Part model, mm, in its own coordinate system. A direction names the side the tool comes from. Round coordinates to 2 decimals unless told otherwise and drop trailing zeros. Write each loop counter-clockwise with the first axis right and the second up, starting at its lowest first coordinate (ties: lowest second). Pieces come first, ordered by that corner, then holes.
```python
from build123d import *

# Parameters (mm, degrees)
BOSS_EXTRUDE1_DEPTH        = 20
SKETCH2_W                  = 22.6
SKETCH2_H                  = 12.7
CUT_EXTRUDE1_DEPTH         = 10
F_2_CLEARANCE_HOLE1_REACH  = 69.082
F_2_CLEARANCE_HOLE1_BORE_R = 1.2192


with BuildPart() as part:
    # Sketch1 → Boss-Extrude1 (new body)
    with BuildSketch(Plane.XY):
        Polygon((1.59, -50), (1.59, -1.59), (38.41, -1.59), (38.41, -50), (40, -50), (40, 0), (0, 0), (0, -50), align=None)
    extrude(amount=BOSS_EXTRUDE1_DEPTH)

    # Sketch2 → Cut-Extrude1 (cut)
    with BuildSketch(Plane(origin=(0, 0, 0), x_dir=(1, 0, 0), z_dir=(0, 1, 0))):
        with Locations((20, -6.35)):
            Rectangle(SKETCH2_W, SKETCH2_H)
    extrude(amount=-CUT_EXTRUDE1_DEPTH, mode=Mode.SUBTRACT)

    # #2 Clearance Hole1 bore → #2 Clearance Hole1 (cut, up to next)
    with BuildSketch(Plane.ZY, mode=Mode.PRIVATE) as f_2_clearance_hole1_sk1:
        with Locations((2.5, -5)):
            Circle(F_2_CLEARANCE_HOLE1_BORE_R)
    f_2_clearance_hole1_tool1 = extrude(f_2_clearance_hole1_sk1.sketch, amount=-F_2_CLEARANCE_HOLE1_REACH, mode=Mode.PRIVATE) & part.part
    # #2 Clearance Hole1 bore → #2 Clearance Hole1 (cut, up to next)
    with BuildSketch(Plane.ZY, mode=Mode.PRIVATE) as f_2_clearance_hole1_sk2:
        with Locations((17.5, -45)):
            Circle(F_2_CLEARANCE_HOLE1_BORE_R)
    f_2_clearance_hole1_tool2 = extrude(f_2_clearance_hole1_sk2.sketch, amount=-F_2_CLEARANCE_HOLE1_REACH, mode=Mode.PRIVATE) & part.part
    add(f_2_clearance_hole1_tool1.solids().sort_by_distance((0, -5, 2.5))[0], mode=Mode.SUBTRACT)
    add(f_2_clearance_hole1_tool2.solids().sort_by_distance((0, -45, 17.5))[0], mode=Mode.SUBTRACT)


solid = part.part
```
Q1. Cut at C-C on z = 2.5. Write the cut outline in (x, y), plus the area to 3 significant figures.
Values follow:
outline: (0, -50) - (1.59, -50) - (1.59, -6.22) - (0, -6.22) - close; (0, -3.78) - (1.59, -3.78) - (1.59, -1.59) - (8.7, -1.59) - (8.7, 0) - (0, 0) - close; (31.3, -1.59) - (38.41, -1.59) - (38.41, -50) - (40, -50) - (40, 0) - (31.3, 0) - close
area: 178 mm2
Q2. Mould opens along X. For faces 4 (the flat face through (1.59, -26, 10)), 5 (the flat face through (40, -25, 10)), 6 (the flat face through (31.3, -1, 6)), 7 (the flat face through (1, -50, 10)) say: +X half, -X half, draft (parallel to the pull), parting line (faces both ways), or undercut.
Values follow:
face 4: undercut
face 5: +X half
face 6: undercut
face 7: draft
Q3. Drop flat-ended pins along their axis: pin 1 (2 mm diameter, centred on y = -45, z = 17.5, fed in from -X); pin 2 (10 mm diameter, centred on x = 21, z = 4, fed in from -Y); pin 3 (1.7 mm diameter, centred on x = 16.5, y = -1, fed in from -Z); pin 4 (10 mm diameter, centred on x = 14.5, z = 9.5, fed in from -Y). Give the stop position or say it passes through.
Values follow:
pin 1: stops at x = 38.41
pin 2: passes through
pin 3: stops at z = 12.7
pin 4: stops at y = -1.59
Q4. Cut at D-D on z = 6.75. Write the cut outline in (x, y), plus the area to 3 significant figures.
Values follow:
outline: (0, -50) - (1.59, -50) - (1.59, -1.59) - (8.7, -1.59) - (8.7, 0) - (0, 0) - close; (31.3, -1.59) - (38.41, -1.59) - (38.41, -50) - (40, -50) - (40, 0) - (31.3, 0) - close
area: 182 mm2
Q5. Which spindle directions (+Z, -Z, +X, -X, +Y, -Y) get a long thin tool onto all of the face, cutting with end or side? Do faces 1 (the cylindrical face through (0.78, -44.18, 16.6)), 2 (the flat face through (38.41, -25, 10)), 3 (the flat face through (20, -1, 12.7)). Say none if no direction does.
Values follow:
face 1: -X
face 2: +Z, -Z, -Y
face 3: -Z, +Y, -Y
Q6. Cut at A-A on z = 17.5. Write the cut outline in (x, y), plus the area to 3 significant figures.
Values follow:
outline: (0, -50) - (1.59, -50) - (1.59, -46.22) - (0, -46.22) - close; (0, -43.78) - (1.59, -43.78) - (1.59, -1.59) - (38.41, -1.59) - (38.41, -50) - (40, -50) - (40, 0) - (0, 0) - close
area: 214 mm2
Q7. Wall check: L1, parallel to Y at x = 0.55, z = 2.5; L2, parallel to Y at x = 1.2, z = 17.5; L3, parallel to X at y = -44.5, z = 19. Give the ranges that are in metal, low to high.
Values follow:
L1: y = -50 to -6.22, -3.78 to 0
L2: y = -50 to -46.22, -43.78 to 0
L3: x = 0 to 1.59, 38.41 to 40
Q8. Cut at B-B on y = -3. Write the cut outline in (x, z).
Values follow:
outline: (0, 0) - (1.59, 0) - (1.59, 20) - (0, 20) - close; (38.41, 0) - (40, 0) - (40, 20) - (38.41, 20) - close
